Autodesk Inventor part; units mm, degrees
ref_plane "YZ Plane" through (0, 0, 0) normal (1, 0, 0) x (0, 1, 0)
ref_plane "XZ Plane" through (0, 0, 0) normal (0, 1, 0) x (-1, 0, 0)
ref_plane "XY Plane" through (0, 0, 0) normal (0, 0, 1) x (1, 0, 0)
sketch "Sketch1" plane through (0, 0, 0) normal (0, 0, 1) x (1, 0, 0)
  line L0 (64.2929, 13) -> (99.1548, 4.0199) construction
  circle A0 centre (64.2929, 13) radius 3 construction
  circle A1 centre (64.2929, 13) radius 4.025 construction
  circle A2 centre (64.2929, 13) radius 7 construction
  arc A3 (102.6474, 8.8986) -> (63.8399, 19.9853) centre (67.7221, -39.8889) ccw construction
  circle A4 centre (99.1548, 4.0199) radius 2.5
  circle A5 centre (99.1548, 4.0199) radius 3.525
  circle A6 centre (99.1548, 4.0199) radius 6
  line L1 (64.2929, 13) -> (98.9408, 0.0186) construction
  line L2 (99.1548, 4.0199) -> (99.1548, -17.9801) construction
  line L3 (99.1548, -17.9801) -> (98.9408, 0.0186) construction
  circle A7 centre (99.1548, -17.9801) radius 10
  circle A8 centre (99.1548, -17.9801) radius 7.025
  line L4 (105.0548, 5.1108) -> (108.9881, -16.162)
  line L5 (93.2548, 5.1108) -> (89.3215, -16.162)
  line L6 (9.3628, -60) -> (214.5663, -60) construction
  arc A9 (95.4028, -0.6623) -> (65.8301, 6.1709) centre (73.5161, -27.9748) ccw construction
  line L7 (99.1548, 4.0199) -> (73.567, -55.2798) construction
  line L8 (99.1548, 4.0199) -> (154.8581, -32.5547) construction
  circle A10 centre (74.7566, -52.523) radius 3
  circle A11 centre (152.3426, -30.903) radius 3
  arc A12 (75.0109, -49.5338) -> (90.7465, -23.3931) centre (76.4523, -32.595) ccw
  arc A13 (109.1059, -16.9921) -> (149.9946, -29.0357) centre (131.9933, -14.7194) ccw
  arc A14 (73.567, -55.2798) -> (154.8581, -32.5547) centre (98.9579, 10.6509) ccw
  circle A15 centre (99.1548, -5.9801) radius 1.25
  circle A16 centre (99.1548, -5.9801) radius 3
  circle A17 centre (99.1548, -5.9801) radius 4.25
  circle A18 centre (99.1548, 4.0199) radius 1.25
  arc A19 (103.9067, -9.1813) -> (101.7399, -9.3536) centre (102.9564, -10.9411) ccw
  arc A20 (96.5698, -9.3536) -> (94.4029, -9.1813) centre (95.3533, -10.9411) ccw
  point P0 (0, 0)
  point P1 (0, 0)
  point P2 (73.6834, -55.3244)
  point P3 (154.7099, -32.7457)
  point P4 (97.1242, -8.1885)
  point P5 (102.5276, -8.5661)
  point P6 (95.7821, -8.5661)
  dimension "d19" = 6
  dimension "d20" = 6
  dimension "d0" = 36
  dimension "d1" = 8.05
  dimension "d2" = 6
  dimension "d3" = 14
  dimension "d4" = 60
  dimension "d5" = 37
  dimension "d6" = 22
  dimension "d7" = 18
  dimension "d8" = 12
  dimension "d9" = 7.05
  dimension "d10" = 20
  dimension "d11" = 14.05
  dimension "d12" = 35
  dimension "d13" = 5
  dimension "d14" = 60
  dimension "d15" = 23.34
  dimension "d17" = 66.6375
  dimension "d18" = 64.5847
  dimension "d21" = 13
  dimension "d23" = 17
  dimension "d29" = 2.5
  dimension "d30" = 6
  dimension "d31" = 8.5
  dimension "d32" = 2.5
  dimension "d43" = 10
  dimension "d44" = 2
  dimension "d45" = 2
  dimension "d46" = 56.711
  dimension "d47" = 23
extrude "Extrusion5" add sketch "Sketch1" against normal blind 5 contours A10 | A7 A20 A17 A19 | A13 A11 A14 A10 A12 A7 | A11
extrude "Extrusion6" add sketch "Sketch1" against normal blind 2 contours A5 | A6 A17 | A6 L4 A7 A17 | A17 A7 A16 A6 | A6 A17 | A6 A17 A7 L5 | A19 A17 A7 | A17 A20 A7 | A7 A16 A17
extrude "Extrusion7" add sketch "Sketch1" against normal blind 3 contours A4 | A16 A7 | A7 A16
chamfer "Chamfer3" distance 1.6 angle 45 2 edges at (97.9048, 4.0199, 0) (97.9048, -5.9801, 0)
sketch "スケッチ5" plane through (0, 0, -5) normal (0, 0, -1) x (-1, 0, 0)
  arc A0 (-149.9946, -29.0357) -> (-154.7099, -32.7457) centre (-152.3426, -30.903) ccw
  arc A1 (-154.7099, -32.7457) -> (-73.6834, -55.3244) centre (-98.9579, 10.6509) ccw
  arc A2 (-73.6834, -55.3244) -> (-75.0109, -49.5338) centre (-74.7566, -52.523) ccw
  arc A3 (-90.7465, -23.3931) -> (-75.0109, -49.5338) centre (-76.4523, -32.595) ccw
  arc A4 (-90.7465, -23.3931) -> (-94.4029, -9.1813) centre (-99.1548, -17.9801) ccw
  arc A5 (-94.4029, -9.1813) -> (-96.5698, -9.3536) centre (-95.3533, -10.9411) ccw
  arc A6 (-101.7399, -9.3536) -> (-96.5698, -9.3536) centre (-99.1548, -5.9801) ccw
  arc A7 (-101.7399, -9.3536) -> (-103.9067, -9.1813) centre (-102.9564, -10.9411) ccw
  arc A8 (-103.9067, -9.1813) -> (-109.1059, -16.9921) centre (-99.1548, -17.9801) ccw
  arc A9 (-149.9946, -29.0357) -> (-109.1059, -16.9921) centre (-131.9933, -14.7194) ccw
  circle A10 centre (-99.1548, -17.9801) radius 7.025
  arc A11 (-133.9095, -41.6513) -> (-108.7322, -28.4278) centre (-131.9933, -14.7194) ccw
  arc A12 (-107.7366, -27.9445) -> (-108.7322, -28.4278) centre (-107.8707, -28.9355) ccw
  line L0 (-107.7366, -27.9445) -> (-106.7456, -28.0786)
  arc A13 (-105.9268, -29.3727) -> (-106.7456, -28.0786) centre (-106.8797, -29.0696) ccw
  arc A14 (-149.9946, -29.0357) -> (-109.1059, -16.9921) centre (-131.9933, -14.7194) ccw
  line L1 (-125.4948, -36.7823) -> (-91.0171, -41.3623) construction
  arc A15 (-90.7465, -23.3931) -> (-75.0109, -49.5338) centre (-76.4523, -32.595) ccw
  line L2 (-125.4948, -36.7823) -> (-99.1548, -17.9801) construction
  line L3 (-99.1548, -17.9801) -> (-91.0171, -41.3623) construction
  line L4 (-99.1548, -17.9801) -> (-114.8496, -67.3215) construction
  line L5 (-105.9268, -29.3727) -> (-113.2937, -52.5329)
  line L6 (-104.7615, -24.3106) -> (-98.127, -25.2082) construction
  arc A16 (-133.9095, -41.6513) -> (-135.1371, -45.326) centre (-134.0514, -43.6463) ccw
  arc A17 (-135.1371, -45.326) -> (-115.702, -53.8625) centre (-98.9579, 10.6509) ccw
  arc A18 (-115.702, -53.8625) -> (-113.2937, -52.5329) centre (-115.1996, -51.9266) ccw
  line L7 (-99.7841, -29.8554) -> (-107.1731, -53.0852)
  arc A19 (-98.697, -29.1675) -> (-99.7841, -29.8554) centre (-98.8311, -30.1585) ccw
  arc A20 (-97.3303, -30.3347) -> (-98.1904, -29.2361) centre (-98.3245, -30.227) ccw
  line L8 (-98.697, -29.1675) -> (-98.1904, -29.2361)
  arc A21 (-97.3303, -30.3347) -> (-86.2751, -51.156) centre (-76.4523, -32.595) ccw
  arc A22 (-86.8471, -54.8905) -> (-86.2751, -51.156) centre (-87.2106, -52.9238) ccw
  arc A23 (-107.1731, -53.0852) -> (-105.4624, -55.6819) centre (-105.2672, -53.6914) ccw
  arc A24 (-105.4624, -55.6819) -> (-86.8471, -54.8905) centre (-98.9579, 10.6509) ccw
  point P0 (0, 0)
  dimension "d57" = 1
  dimension "d58" = 1
  dimension "d59" = 4
  dimension "d60" = 73.669
  dimension "d61" = 36.835
  dimension "d62" = 3
  dimension "d63" = 1
  dimension "d64" = 4
  dimension "d66" = 2
  dimension "d67" = 4
  dimension "d68" = 2
  dimension "d70" = 3
  dimension "d71" = 1
  dimension "d72" = 1
  dimension "d73" = 4
  dimension "d74" = 4
  dimension "d75" = 2
  dimension "d76" = 2
  dimension "d77" = 4
extrude "押し出し8" cut sketch "スケッチ5" against normal blind 1.2 contours A11 A12 L0 A13 L5 A18 A17 A16 | A19 L8 A20 A21 A22 A24 A23 L7
properties part number "ヘッケン" material "ポリカーボネート、クリア"
Build history of the part. All positions in model axes, mm. A direction names the side the tool comes from. Coordinates: 2 decimals unless noted, no trailing zeros. Order: outer loops, then holes, each group sorted by start corner. A loop starts at its lowest first (then second) coordinate and runs counter-clockwise, first axis right, second up. Notation, with made-up numbers: (4, -31.5) - (47, -31.5) arc R13 ccw to (47, -8.5) - close; hole circle Ø11 at (32, 53.25). An arc over 180 degrees is marked (long way). Put each result on its own line as item: value.
1. Saw through at A-A (y = -1). Write the cut outline in (x, z).
Answer sheet:
outline: (92.12, -2) - (106.18, -2) - (106.18, 0) - (92.12, 0) - close
2. Probe line 1 along X through (y, z) = (-30.5, -2.6); line 2 along Y through (x, z) = (105.5, -3.2); line 3 along X through (y, z) = (-35, -2.7). List the from-to ranges inside material, lowest first. Write a range as [from, to].
Answer sheet:
line 1: x = [93.32, 115.26], [148.73, 155.32]
line 2: y = [-59.7, -20.99], [-14.97, -10.25]
line 3: x = [93.28, 121.14], [142.84, 152.88]
3. Pull direction Y, two halves, no side cores. Call faces 3 (the face through (107, -5.4, -1)), 4 (the face through (89.187, -17.178, -3.021)), 5 (the face through (117.25, -57.59, -2.46)): pulls with the +Y half, pulls with the -Y half, needs draft (parallel to the pull), parting line crosses it, or undercut.
Answer sheet:
face 3: pulls with the +Y half
face 4: undercut
face 5: pulls with the -Y half
4. Drop flat-ended pins along their axis: P1, Ø3, axis at x = 131, z = -1.5, coming from the -Y side; P2, Ø6, axis at x = 98.5, y = -1, coming from the -Z side. Give the stop position or say it passes through.
Answer sheet:
P1: stops at y = -53.06
P2: stops at z = -3
5. Tool access for faces 1 (the face through (103.427, -41.308, -4.408)), 2 (the face through (100.31, 3.54, -2.29)): list every direction of +Z, -Z, +X, -X, +Y, -Y with a clear straight run to the whole face (end or side of a thin tool).
Answer sheet:
face 1: -Z
face 2: +Z, -Z
